Design review of the part shown in the three views and the two pictorial views. Dimensions are in mm from the part's minimum x, y and z. Round coordinates to 2 decimals unless told otherwise and drop trailing zeros. Order: outer loops, then holes, each group sorted by start corner. A loop starts at its lowest first (then second) coordinate and runs counter-clockwise, first axis right, second up.
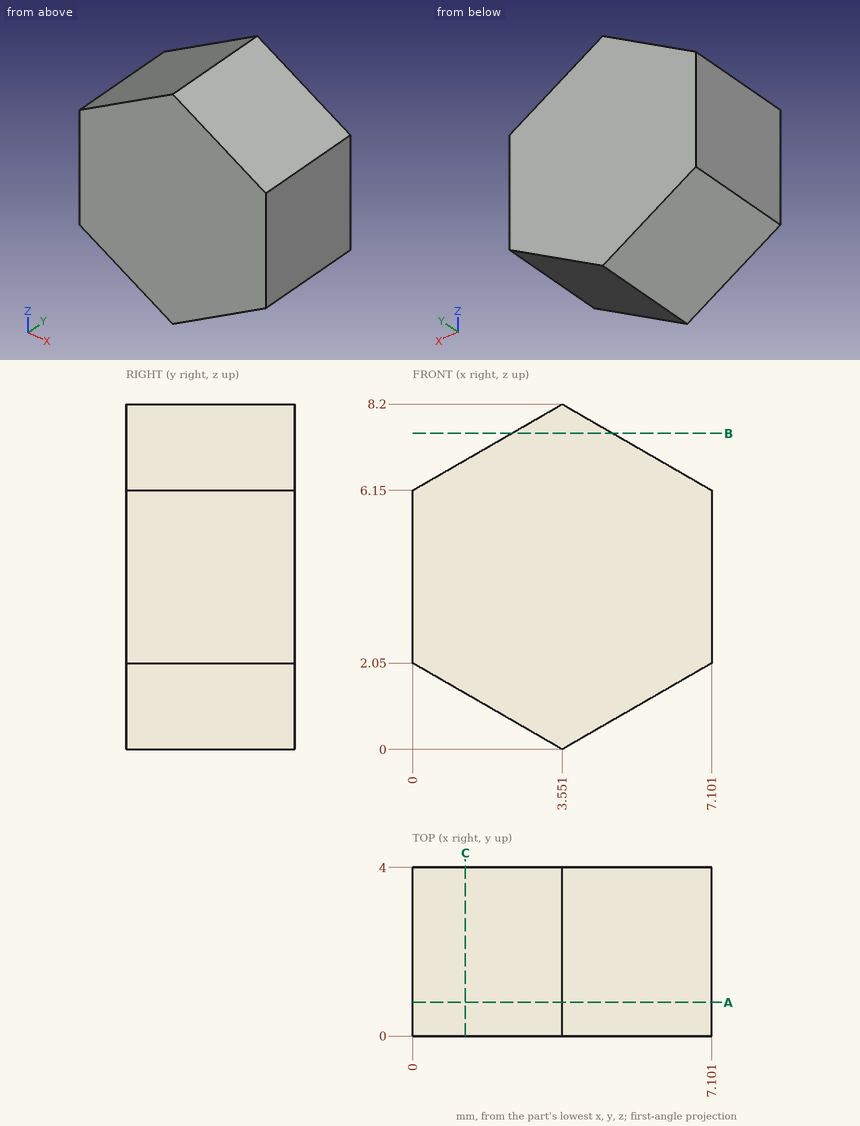
1) Take a section at B-B on z = 7.5. Give the boundary of the cut face in (x, y).
Results:
outline: (2.34, 0) - (4.76, 0) - (4.76, 4) - (2.34, 4) - close
2) Take a section at C-C on x = 1.25. Give the boundary of the cut face in (y, z).
Results:
outline: (0, 1.33) - (4, 1.33) - (4, 6.87) - (0, 6.87) - close
3) To check wall thickness, follow line 1 along Z through (x, y) = (5.5, 1.65) (1 decimal); line 2 along Z through (x, y) = (2.5, 2.75) (1 decimal); line 3 along X through (y, z) = (3.15, 6.25) (1 decimal). State the ranges of each line that lie inside material, in increasing order.
Results:
line 1: z = 1.1 to 7.1
line 2: z = 0.6 to 7.6
line 3: x = 0.2 to 6.9
4) Take a section at A-A on y = 0.8. Give the boundary of the cut face in (x, z).
Results:
outline: (0, 2.05) - (3.55, 0) - (7.1, 2.05) - (7.1, 6.15) - (3.55, 8.2) - (0, 6.15) - close
